Check sheet for the modelled part. Datum: model origin and axes. Units: mm. Give positions to 0.01 mm unless a question says otherwise; leave off trailing zeros. Order: outer loops, then holes, each group sorted by start corner. A loop starts at its lowest first (then second) coordinate and runs counter-clockwise, first axis right, second up.
Item 1: Material ranges on line 1 along Y through (x, z) = (10.5, 3.75); line 2 along Y through (x, z) = (2, 2.75); line 3 along Z through (x, y) = (-24, 4.3), recorded low to high.
Item 2: Sectioned sample at A-A on x = -12. Record the boundary of the cut face in (y, z), and give its area (3 significant figures).
Item 3: Gauge pin test, flat ends, axial feed: P1, Ø2, axis at y = 7, z = 1.5, coming from the +X side; P2, Ø1.5, axis at x = 10, y = 5.5, coming from the -Z side. Record the tip position at first contact, or that the pin passes through.
Item 4: Sectioned sample at B-B on y = 7.6. Record the boundary of the cut face in (x, z).
from build123d import *

# Parameters (mm, degrees)
SKETCH1_W               = 50.8
SKETCH1_H               = 3.464243611
BASE_EXTRUDE_DEPTH      = 50.8
BOSS_EXTRUDE1_DEPTH     = 19.05
BOSS_REVOLVE1_ANGLE     = 90
FILLET1_R               = 3.048
CUT_EXTRUDE2_DEPTH      = 58.490562181
CUT_EXTRUDE2_DEPTH_BACK = 58.490562181
SKETCH5_W               = 50.8
SKETCH5_H               = 3.464243611
CUT_EXTRUDE1_DEPTH      = 106.06310615


with BuildPart() as part:
    # Sketch1 → Base-Extrude (new, symmetric)
    with BuildSketch(Plane(origin=(0, 0, 0), x_dir=(0, 0, -1), z_dir=(1, 0, 0))):
        with Locations((0, 1.732121806)):
            Rectangle(SKETCH1_W, SKETCH1_H)
    extrude(amount=BASE_EXTRUDE_DEPTH, both=True)

    # Sketch3 → Boss-Extrude1 (add, symmetric)
    with BuildSketch(Plane(origin=(0, 4.664955708, 2.581196581), x_dir=(0, 0, 1), z_dir=(1, 0, 0))):
        with BuildLine():
            Line((-4.547008547, 1.200712097), (-4.547008547, -4.243732347))
            ThreePointArc((-4.547008547, -4.243732347), (-0.697204961, -2.649091489), (0.897435897, 1.200712097))
            Line((0.897435897, 1.200712097), (-4.547008547, 1.200712097))
        make_face()
    extrude(amount=BOSS_EXTRUDE1_DEPTH, both=True)

    # Sketch4 → Boss-Revolve1 (revolve)
    with BuildSketch(Plane.ZY.offset(19.05)):
        with BuildLine():
            Line((-1.965811966, 3.464243611), (3.478632479, 3.464243611))
            ThreePointArc((3.478632479, 3.464243611), (1.883991621, 7.314047197), (-1.965811966, 8.908688055))
            Line((-1.965811966, 8.908688055), (-1.965811966, 3.464243611))
        make_face()
    boss_revolve1 = revolve(axis=Axis((-19.05, 3.464243611, -1.965811966), (0, -1, 0)), revolution_arc=BOSS_REVOLVE1_ANGLE)

    # Mirror1: Boss-Revolve1 across plane
    add(boss_revolve1.mirror(Plane(origin=(0, 0, 0), x_dir=(0, 0, 1), z_dir=(1, 0, 0))))

    # Fillet1
    fillet1_edges = [part.edges().sort_by_distance(p)[0] for p in [
        (0, 3.464243611, 3.478632479),
        (-22.899803586, 3.464243611, 1.883991621),
        (22.899803586, 3.464243611, 1.883991621),
    ]]
    fillet(fillet1_edges, radius=FILLET1_R)

    # Sketch7 → Cut-Extrude2 (cut, two sides: drawn at the far end of the back side and taken through both)
    with BuildSketch(Plane(origin=(0, 0, 0), x_dir=(0, 0, -1), z_dir=(1, 0, 0)).offset(-CUT_EXTRUDE2_DEPTH_BACK)):
        with BuildLine():
            Line((1.965811966, 3.464243611), (-0.335109681, 8.398586007))
            ThreePointArc((-0.335109681, 8.398586007), (0.787418512, 8.779632983), (1.965811966, 8.908688055))
            Line((1.965811966, 8.908688055), (1.965811966, 3.464243611))
        make_face()
    extrude(amount=CUT_EXTRUDE2_DEPTH + CUT_EXTRUDE2_DEPTH_BACK, mode=Mode.SUBTRACT)

    # Sketch5 → Cut-Extrude1 (cut, through all)
    with BuildSketch(Plane.ZY.offset(50.8)):
        with Locations((0, 1.732121806)):
            Rectangle(SKETCH5_W, SKETCH5_H)
    extrude(amount=-CUT_EXTRUDE1_DEPTH, mode=Mode.SUBTRACT)


solid = part.part
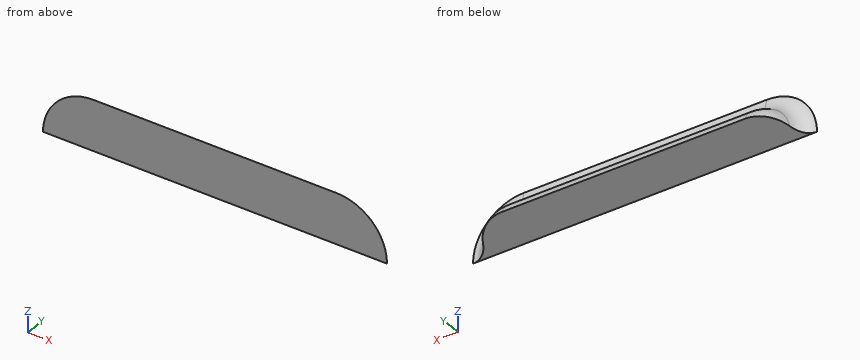
Report:
1. line 1: y = 3.46 to 4.41
1. line 2: y = 3.46 to 6.19
1. line 3: z = -1.58 to 1.11
2. outline: (3.46, -1.97) - (8.4, 0.34) arc R5.44 ccw to (5.42, 3.12) arc R3.05 cw to (3.46, 5.96) - close
2. area: 17.9 mm2
3. P1: stops at x = 22.8
3. P2: stops at z = -1.37
4. outline: (-22.02, -0.04) - (22.02, -0.04) arc R3.54 ccw to (19.05, 1.58) - (-19.05, 1.58) arc R3.54 ccw to start
